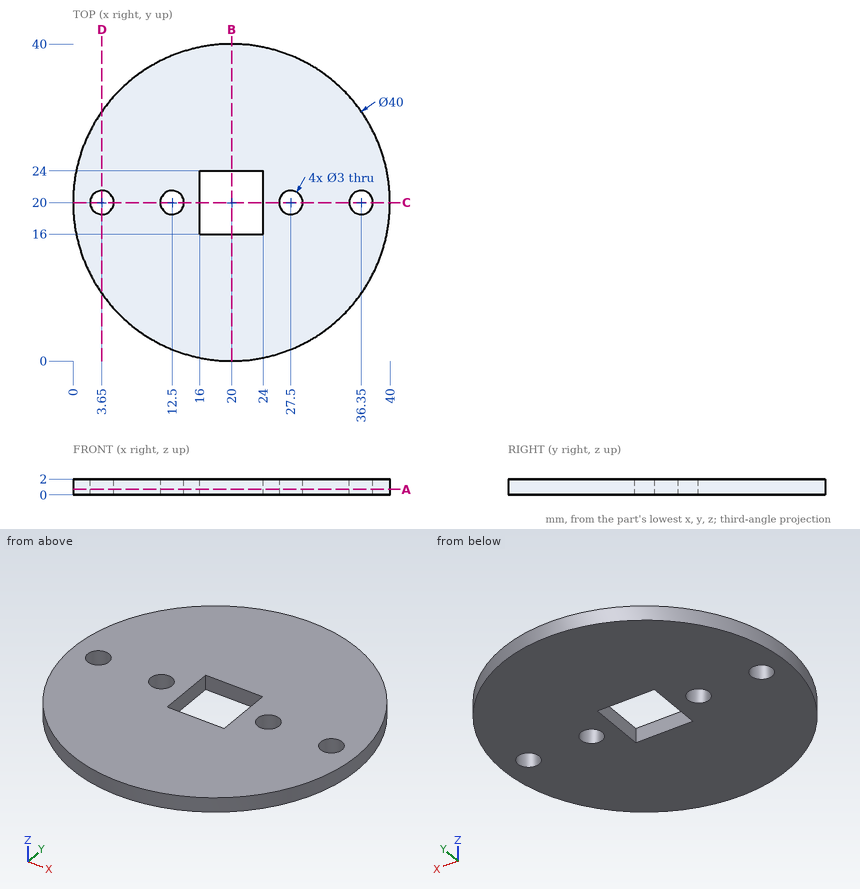
Job drawing, mm, ordinate dimensions from the low corner. One solid piece. Round coordinates to 2 decimals unless told otherwise and drop trailing zeros. Loops run counter-clockwise (first coordinate to the right, second up) from the corner with the lowest first, then second, coordinate; pieces in that order, holes last.
Item 1: Cut at D-D, the plane x = 3.65. Give the cut face in (y, z), then the cut area to 3 significant figures.
Item 2: Drop flat-ended pins along their axis: P1, Ø1.5, axis at x = 16.5, y = 20, coming from the +Z side; P2, Ø0.6, axis at y = 20.5, z = 1, coming from the +X side; P3, Ø0.6, axis at y = 19, z = 1, coming from the -X side. Give the stop position or say it passes through.
Item 3: Drill centre lines: line 1 (Y direction, x = 20.5, z = 0.15); line 2 (X direction, y = 16.5, z = 0.35); line 3 (Y direction, x = 27.5, z = 1.65). Where is each one in solid material? Low to high.
Item 4: Cut at A-A, the plane z = 0.7. Give the cut face in (x, y).
Item 5: Cut at B-B, the plane x = 20. Give the cut face in (y, z).
Item 6: Cut at C-C, the plane y = 20. Give the cut face in (x, z), then the cut area to 3 significant figures.
A:
1. outline: (8.48, 0) - (18.5, 0) - (18.5, 2) - (8.48, 2) - close; (21.5, 0) - (31.52, 0) - (31.52, 2) - (21.5, 2) - close
1. area: 40.1 mm2
2. P1: stops at z = 2
2. P2: stops at x = 40
2. P3: stops at x = 0.01
3. line 1: y = 0.01 to 16, 24 to 39.99
3. line 2: x = 0.31 to 16, 24 to 39.69
3. line 3: y = 1.46 to 18.5, 21.5 to 38.54
4. outline: circle Ø40 at (20, 20); hole circle Ø3 at (3.65, 20); hole circle Ø3 at (12.5, 20); hole (16, 16) - (24, 16) - (24, 24) - (16, 24) - close; hole circle Ø3 at (27.5, 20); hole circle Ø3 at (36.35, 20)
5. outline: (0, 0) - (16, 0) - (16, 2) - (0, 2) - close; (24, 0) - (40, 0) - (40, 2) - (24, 2) - close
6. outline: (0, 0) - (2.15, 0) - (2.15, 2) - (0, 2) - close; (5.15, 0) - (11, 0) - (11, 2) - (5.15, 2) - close; (14, 0) - (16, 0) - (16, 2) - (14, 2) - close; (24, 0) - (26, 0) - (26, 2) - (24, 2) - close; (29, 0) - (34.85, 0) - (34.85, 2) - (29, 2) - close; (37.85, 0) - (40, 0) - (40, 2) - (37.85, 2) - close
6. area: 40.0 mm2
